Build history of the part. All positions in model axes, mm. Face numbers are marked on the shaded views. Round coordinates to 2 decimals unless told otherwise and drop trailing zeros. Order: outer loops, then holes, each group sorted by start corner. A loop starts at its lowest first (then second) coordinate and runs counter-clockwise, first axis right, second up. Notation, with made-up numbers: (85.5, -1.75) -> (98.5, -1.75) arc R22 cw to (98.5, 19.25) -> close; hole circle Ø6 at (50.25, 29.25). An arc over 180 degrees is marked (long way). Answer as a JSON object with one key per item and string values.
from build123d import *

# Parameters (mm, degrees)
SKETCH1_R           = 10
SKETCH1_R_2         = 4.5
BOSS_EXTRUDE1_DEPTH = 20
SKETCH2_R           = 1
CUT_EXTRUDE1_DEPTH  = 2


with BuildPart() as part:
    # Sketch1 → Boss-Extrude1 (new body)
    with BuildSketch(Plane(origin=(0, 0, 0), x_dir=(1, 0, 0), z_dir=(0, 1, 0))):
        with Locations(Location((0, 0, 0), (0, 0, 270))):
            Circle(SKETCH1_R)
        with Locations(Location((0, 0, 0), (0, 0, 270))):
            Circle(SKETCH1_R_2, mode=Mode.SUBTRACT)
    extrude(amount=BOSS_EXTRUDE1_DEPTH)

    # Sketch2 → Cut-Extrude1 (cut)
    with BuildSketch(Plane.XZ):
        with Locations(Location((-7.25, 0, 0), (0, 0, 270))):
            Circle(SKETCH2_R)
        with Locations(Location((-6.532024292, 3.145657109, 0), (0, 0, 270))):
            Circle(SKETCH2_R)
        with Locations(Location((-4.520301063, 5.668278248, 0), (0, 0, 270))):
            Circle(SKETCH2_R)
        with Locations(Location((-1.613276771, 7.068227363, 0), (0, 0, 270))):
            Circle(SKETCH2_R)
        with Locations(Location((1.613276771, 7.068227363, 0), (0, 0, 270))):
            Circle(SKETCH2_R)
        with Locations(Location((4.520301063, 5.668278248, 0), (0, 0, 270))):
            Circle(SKETCH2_R)
        with Locations(Location((6.532024292, 3.145657109, 0), (0, 0, 270))):
            Circle(SKETCH2_R)
        with Locations(Location((7.25, 0, 0), (0, 0, 270))):
            Circle(SKETCH2_R)
        with Locations(Location((6.532024292, -3.145657109, 0), (0, 0, 270))):
            Circle(SKETCH2_R)
        with Locations(Location((4.520301063, -5.668278248, 0), (0, 0, 270))):
            Circle(SKETCH2_R)
        with Locations(Location((1.613276771, -7.068227363, 0), (0, 0, 270))):
            Circle(SKETCH2_R)
        with Locations(Location((-1.613276771, -7.068227363, 0), (0, 0, 270))):
            Circle(SKETCH2_R)
        with Locations(Location((-4.520301063, -5.668278248, 0), (0, 0, 270))):
            Circle(SKETCH2_R)
        with Locations(Location((-6.532024292, -3.145657109, 0), (0, 0, 270))):
            Circle(SKETCH2_R)
    extrude(amount=-CUT_EXTRUDE1_DEPTH, mode=Mode.SUBTRACT)


solid = part.part
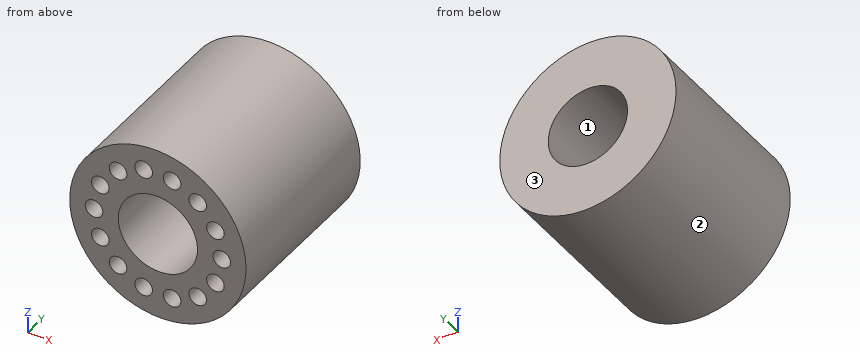
1) Cut at C-C, the plane y = 15.75. Give the cut face in (x, z), plus the area to 3 significant figures.
Checked values:
{"outline": "circle Ø20 at (0, 0); hole circle Ø9 at (0, 0)", "area": "251 mm²"}
2) Cut at D-D, the plane x = 7.25. Give the cut face in (y, z), plus the area to 3 significant figures.
Checked values:
{"outline": "(0, -6.89) -> (20, -6.89) -> (20, 6.89) -> (0, 6.89) -> (0, 3.84) -> (2, 3.84) -> (2, 2.45) -> (0, 2.45) -> (0, 1) -> (2, 1) -> (2, -1) -> (0, -1) -> (0, -2.45) -> (2, -2.45) -> (2, -3.84) -> (0, -3.84) -> close", "area": "266 mm²"}
3) Flat gauge pins, fed straight in: pin 1 Ø6 at (x, y) = (6.5, 16.5) entering from +Z; pin 2 Ø4 at (x, y) = (-7.5, 8.5) entering from -Z; pin 3 Ø1 at (x, z) = (-4.5, -5.5) entering from -Y. Where does each tip first touch, or does it go through?
Checked values:
{"pin 1": "stops at z = 9.37", "pin 2": "stops at z = -8.35", "pin 3": "stops at y = 2"}
4) Pull direction Z, two halves, no side cores. Call the marked faces 1, 2 and 3: pulls with the +Z half, pulls with the -Z half, needs draft (parallel to the pull), parting line crosses it, or undercut.
Checked values:
{"face 1": "undercut", "face 2": "parting line crosses it", "face 3": "needs draft"}
5) Probe L1, parallel to X at y = 3.75, z = -2; L2, parallel to X at y = 7.5, z = 0; L3, parallel to Z at x = 2.5, y = 16. List the from-to ranges inside material, lowest first. Write a range as from..to.
Checked values:
{"L1": "x = -9.8..-4.03, 4.03..9.8", "L2": "x = -10..-4.5, 4.5..10", "L3": "z = -9.68..-3.74, 3.74..9.68"}
6) Cut at A-A, the plane x = 0. Give the cut face in (y, z).
Checked values:
{"outline": "(0, -10) -> (20, -10) -> (20, -4.5) -> (0, -4.5) -> close; (0, 4.5) -> (20, 4.5) -> (20, 10) -> (0, 10) -> close"}
7) Cut at B-B, the plane z = 0. Give the cut face in (x, y), plus the area to 3 significant figures.
Checked values:
{"outline": "(-10, 0) -> (-8.25, 0) -> (-8.25, 2) -> (-6.25, 2) -> (-6.25, 0) -> (-4.5, 0) -> (-4.5, 20) -> (-10, 20) -> close; (4.5, 0) -> (6.25, 0) -> (6.25, 2) -> (8.25, 2) -> (8.25, 0) -> (10, 0) -> (10, 20) -> (4.5, 20) -> close", "area": "212 mm²"}
